Design review of the part built by this model. Coordinates are the model's own, in mm. A direction names the side the tool comes from. Give positions to 0.01 mm unless a question says otherwise; leave off trailing zeros. Order: outer loops, then holes, each group sorted by start corner. A loop starts at its lowest first (then second) coordinate and runs counter-clockwise, first axis right, second up.
```python
from build123d import *

# Parameters (mm, degrees)
SKETCH001_R      = 1.75
PAD_DEPTH        = 2
FILLET_R         = 1.98
SKETCH002_R      = 6
SKETCH002_R_2    = 5
PAD001_DEPTH     = 10
HOLE_D           = 3.4
HOLE_CBORE_D     = 6.1
HOLE_CBORE_DEPTH = 3.4
SKETCH004_R      = 1.7
PAD002_DEPTH     = 0.2


with BuildPart() as part:
    # Sketch001 → Pad (new body)
    with BuildSketch(Plane.XY):
        Polygon((-99.5, 65), (-89.5, 65), (-89.5, 55), (89.5, 55), (89.5, 65), (99.5, 65), (99.5, -65), (89.5, -65), (89.5, -55), (-89.5, -55), (-89.5, -65), (-99.5, -65), align=None)
        with Locations((-94.5, 60)):
            Circle(SKETCH001_R, mode=Mode.SUBTRACT)
        with Locations((94.5, 60)):
            Circle(SKETCH001_R, mode=Mode.SUBTRACT)
        with Locations((-94.5, -60)):
            Circle(SKETCH001_R, mode=Mode.SUBTRACT)
        with Locations((94.5, -60)):
            Circle(SKETCH001_R, mode=Mode.SUBTRACT)
        Polygon((-77.5, 45), (28.5, 45), (28.5, 30), (32.5, 30), (32.5, -35), (28.5, -35), (28.5, -45), (-77.5, -45), (-77.5, -35), (-87.5, -35), (-87.5, 30), (-77.5, 30), align=None, mode=Mode.SUBTRACT)
        Polygon((48.5, 45), (87.5, 45), (87.5, -45), (48.5, -45), (48.5, -35), (44.5, -35), (44.5, 30), (48.5, 30), align=None, mode=Mode.SUBTRACT)
    extrude(amount=PAD_DEPTH)

    # Fillet
    fillet_edges = [part.edges().sort_by_distance(p)[0] for p in [
        (-89.5, -65, 1),
        (-99.5, -65, 1),
        (-89.5, -55, 1),
        (48.5, 30, 1),
        (48.5, 45, 1),
        (87.5, 45, 1),
        (-77.5, 30, 1),
        (-77.5, 45, 1),
        (-89.5, 55, 1),
        (-89.5, 65, 1),
        (-99.5, 65, 1),
        (28.5, 45, 1),
        (28.5, 30, 1),
        (32.5, 30, 1),
        (32.5, -35, 1),
        (28.5, -35, 1),
        (89.5, 55, 1),
        (89.5, 65, 1),
        (99.5, 65, 1),
        (99.5, -65, 1),
        (89.5, -65, 1),
        (89.5, -55, 1),
        (28.5, -45, 1),
        (-77.5, -45, 1),
        (-77.5, -35, 1),
        (-87.5, -35, 1),
        (-87.5, 30, 1),
        (44.5, -35, 1),
        (48.5, -35, 1),
        (48.5, -45, 1),
        (87.5, -45, 1),
        (44.5, 30, 1),
    ]]
    fillet(fillet_edges, radius=FILLET_R)

    # Sketch002 → Pad001 (join)
    with BuildSketch(Plane.XY.offset(2)):
        with Locations((-87.5, 40)):
            Circle(SKETCH002_R)
        with Locations((38.5, 40)):
            Circle(SKETCH002_R)
        with Locations((38.5, -45)):
            Circle(SKETCH002_R)
        with Locations((-87.5, -45)):
            Circle(SKETCH002_R)
        with Locations((92, -45)):
            Circle(SKETCH002_R_2)
        with Locations((92, 45)):
            Circle(SKETCH002_R_2)
    extrude(amount=PAD001_DEPTH)

    # Hole (through all)
    with Locations(Plane(origin=(0, 0, 0), x_dir=(1, 0, 0), z_dir=(0, 0, -1))):
        with Locations((-87.5, -40), (38.5, -40), (38.5, 45), (-87.5, 45)):
            CounterBoreHole(HOLE_D / 2, HOLE_CBORE_D / 2, HOLE_CBORE_DEPTH)

    # Sketch004 → Pad002 (join)
    with BuildSketch(Plane.XY.offset(3.4)):
        with Locations((-87.5, 40)):
            Circle(SKETCH004_R)
        with Locations((38.5, 40)):
            Circle(SKETCH004_R)
        with Locations((38.5, -45)):
            Circle(SKETCH004_R)
        with Locations((-87.5, -45)):
            Circle(SKETCH004_R)
    extrude(amount=PAD002_DEPTH)


solid = part.part
```
1. Draft analysis for pull direction Y (two halves, no side actions). For faces 1 (the face through (33.74, -48.65, 6.93)), 2 (the face through (92, -45, 12)), state which applies: pulls with the +Y half, pulls with the -Y half, needs draft (parallel to the pull), parting line crosses it, or undercut.
Recorded:
face 1: undercut
face 2: needs draft
2. Machinability: for faces 3 (the face through (-88, 40, 3.4)), 4 (the face through (33.74, 36.35, 6.93)), 5 (the face through (-86.25, 41.42, 12)), which of the approach directions +Z, -Z, +X, -X, +Y, -Y give a long, thin tool a straight path to every point of the face, cutting with its end or side? Answer none if there is none.
Recorded:
face 3: -Z
face 4: +Z
face 5: +Z, +X, -X, +Y, -Y
3. For pin 1 (3 mm diameter, centred on x = 38.5, y = -45, fed in from -Z); pin 2 (1.5 mm diameter, centred on x = -17.5, z = 2, fed in from -Y); pin 3 (1 mm diameter, centred on y = -24.5, z = 4, fed in from -X); pin 4 (3 mm diameter, centred on y = -38.5, z = 4.5, fed in from -X), all flat-tipped, find the tip position at first contact; note any pin that passes through.
Recorded:
pin 1: stops at z = 3.4
pin 2: stops at y = -55
pin 3: passes through
pin 4: stops at x = -90.82
4. Take a section at A-A (z = 8). State how many separate pieces and enclosed holes the cut face has, then the cut area to 3 significant figures.
Recorded:
separate pieces: 6
enclosed holes: 4
area: 573 mm2
5. For line 1 along X through (y, z) = (40, 1.5); line 2 along Y through (x, z) = (94.5, 1.65); line 3 along X through (y, z) = (24, 1.5), list the stretches that pass through material, from the lowest coordinate up.
Recorded:
line 1: x = -99.5 to -90.55, -84.45 to -77.5, 28.5 to 35.45, 41.55 to 48.5, 87.5 to 99.5
line 2: y = -65 to -61.75, -58.25 to 58.25, 61.75 to 65
line 3: x = -99.5 to -87.5, 32.5 to 44.5, 87.5 to 99.5
6. Take a section at B-B (y = 8.5). State the section outline as (x, z) points, then the cut area to 3 significant figures.
Recorded:
outline: (-99.5, 0) - (-87.5, 0) - (-87.5, 2) - (-99.5, 2) - close; (32.5, 0) - (44.5, 0) - (44.5, 2) - (32.5, 2) - close; (87.5, 0) - (99.5, 0) - (99.5, 2) - (87.5, 2) - close
area: 72.0 mm2
7. Take a section at C-C (x = 72.5). State the section outline as (y, z) points.
Recorded:
outline: (-55, 0) - (-45, 0) - (-45, 2) - (-55, 2) - close; (45, 0) - (55, 0) - (55, 2) - (45, 2) - close
